Read the model definition and answer for the solid it produces. Units are mm, in the model's axes. Face numbers are marked on the shaded views. A direction names the side the tool comes from. Coordinates: 2 decimals unless noted, no trailing zeros. Loops run counter-clockwise (first coordinate to the right, second up) from the corner with the lowest first, then second, coordinate; pieces in that order, holes last. Notation, with made-up numbers: (71.5, -13.5) -> (122.5, -13.5) arc R23 cw to (122.5, -2.5) -> close; hole circle Ø6 at (59.25, -3.5). An arc over 180 degrees is marked (long way). Answer as a JSON object with one key per item and string values. Group by question number.
Q1. The part is cut by section C-C on y = -133. Write down the section's boundary in (x, z), and give its area (3 significant figures).
Q2. For the marked faces 3, 4 and 5, determine the directions among +Z, -Z, +X, -X, +Y, -Y from which every point of the face is accessible in a straight line to the end or side of a thin tool.
Q3. The part is cut by section B-B on x = 72. Write down the section's boundary in (y, z), and give its area (3 significant figures).
Q4. The part is cut by section A-A on z = 306. Write down the section's boundary in (x, y), and give its area (3 significant figures).
Q5. The part is cut by section D-D on x = -212. Write down the section's boundary in (y, z), and give its area (3 significant figures).
Q6. Straight lines are drawn through the part: line 1 along X through (y, z) = (211, 206.5); line 2 along Y through (x, z) = (-226.5, 29.5); line 3 along Z through (x, y) = (177, -220.5). For each, find the intervals that lie inside material, in ascending order. Write a range as [from, to].
Q7. Each of these flat-tipped pins is pushed along its axis until it touches: P1, Ø15, axis at x = 25.5, z = 36.5, coming from the +Y side; P2, Ø20, axis at x = 221, z = 232.5, coming from the +Y side; P3, Ø3, axis at x = 0, y = -58, coming from the -Z side; P4, Ø16, axis at x = -13.5, y = -205, coming from the +Z side. Where does it stop, or does it pass through?
Q8. Determine the mould class of the marked faces 1 and 2 for opening direction X: released by +X, released by -X, zero draft, split by the parting line, or undercut.
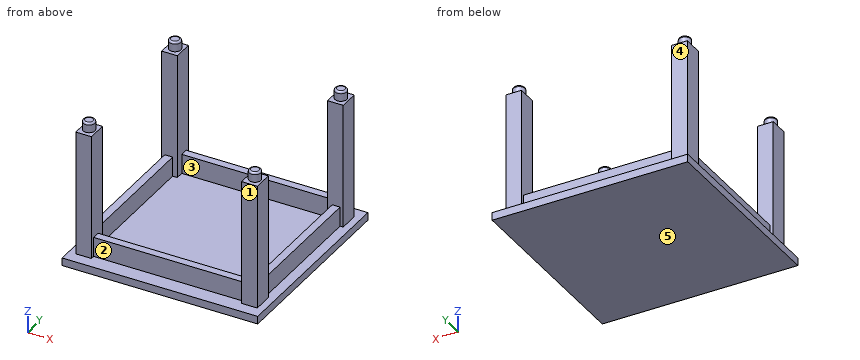
from build123d import *

# Parameters (mm, degrees)
F0_W     = 500
F0_H     = 500
F1_DEPTH = 20
F2_W     = 40
F2_H     = 50
F3_DEPTH = 320
F4_W     = 384
F4_H     = 20
F4_W_2   = 20
F4_H_2   = 340
F5_DEPTH = 50
F7_R     = 15
F8_DEPTH = 25
F9_R     = 5


with BuildPart() as f1:
    # F0 (on Top) → F1 (new body)
    with BuildSketch(Plane.XY):
        Rectangle(F0_W, F0_H)
    extrude(amount=F1_DEPTH)

    # F2 (on face) → F3 (join)
    with BuildSketch(Plane.XY.offset(20)):
        with Locations((212, 195)):
            Rectangle(F2_W, F2_H)
        with Locations((-212, -195)):
            Rectangle(F2_W, F2_H)
        with Locations((212, -195)):
            Rectangle(F2_W, F2_H)
        with Locations((-212, 195)):
            Rectangle(F2_W, F2_H)
    extrude(amount=F3_DEPTH)

    # F4 (on face) → F5 (join)
    with BuildSketch(Plane.XY.offset(20)):
        with Locations((0, -200)):
            Rectangle(F4_W, F4_H)
        Polygon((-192, 199.430282), (-192, 190), (192, 190), (192, 195), (192, 210), (-192, 210), align=None)
        with Locations((214.009886, 0)):
            Rectangle(F4_W_2, F4_H_2)
        with Locations((-214.009886, 0)):
            Rectangle(F4_W_2, F4_H_2)
    extrude(amount=F5_DEPTH)

    # F7 (on face) → F8 (join)
    with BuildSketch(Plane.XY.offset(340)):
        with Locations((212, 195)):
            Circle(F7_R)
        with Locations((-212, 195)):
            Circle(F7_R)
        with Locations((212, -195)):
            Circle(F7_R)
        with Locations((-212, -195)):
            Circle(F7_R)
    extrude(amount=F8_DEPTH)

    # F9
    f9_edges = [f1.edges().sort_by_distance(p)[0] for p in [
        (197, 195, 365),
        (197, -195, 365),
        (-227, -195, 365),
        (-227, 195, 365),
    ]]
    fillet(f9_edges, radius=F9_R)


solid = f1.part
Final values:
{
 "1": {"outline": "(-250, 0) -> (250, 0) -> (250, 20) -> (224.01, 20) -> (224.01, 70) -> (204.01, 70) -> (204.01, 20) -> (-204.01, 20) -> (-204.01, 70) -> (-224.01, 70) -> (-224.01, 20) -> (-250, 20) -> close", "area": "12,000 mm2"},
 "2": {"face 3": "+Z", "face 4": "+Z, +X, -X, +Y", "face 5": "-Z, +X, -X, +Y, -Y"},
 "3": {"outline": "(-250, 0) -> (250, 0) -> (250, 20) -> (210, 20) -> (210, 70) -> (190, 70) -> (190, 20) -> (-190, 20) -> (-190, 70) -> (-210, 70) -> (-210, 20) -> (-250, 20) -> close", "area": "12,000 mm2"},
 "4": {"outline": "(-232, -220) -> (-192, -220) -> (-192, -170) -> (-232, -170) -> close; (-232, 170) -> (-192, 170) -> (-192, 220) -> (-232, 220) -> close; (192, -220) -> (232, -220) -> (232, -170) -> (192, -170) -> close; (192, 170) -> (232, 170) -> (232, 220) -> (192, 220) -> close", "area": "8,000 mm2"},
 "5": {"outline": "(-250, 0) -> (250, 0) -> (250, 20) -> (220, 20) -> (220, 340) -> (210, 340) -> (210, 360) arc R5 ccw to (205, 365) -> (185, 365) arc R5 ccw to (180, 360) -> (180, 340) -> (170, 340) -> (170, 70) -> (-170, 70) -> (-170, 340) -> (-180, 340) -> (-180, 360) arc R5 ccw to (-185, 365) -> (-205, 365) arc R5 ccw to (-210, 360) -> (-210, 340) -> (-220, 340) -> (-220, 20) -> (-250, 20) -> close", "area": "60,500 mm2"},
 "6": {"line 1": "x = [-232, -192], [192, 232]", "line 2": "y = [-220, -170], [170, 220]", "line 3": "z = [0, 20]"},
 "7": {"P1": "stops at y = 210", "P2": "stops at y = 220", "P3": "stops at z = 0", "P4": "stops at z = 70"},
 "8": {"face 1": "zero draft", "face 2": "undercut"}
}
